Source: CAD feature listing. Evaluate the final solid. Frame: model axes, mm. A direction names the side the tool comes from. Round coordinates to 2 decimals unless told otherwise and drop trailing zeros. Write each loop counter-clockwise with the first axis right and the second up, starting at its lowest first coordinate (ties: lowest second). Pieces come first, ordered by that corner, then holes. Notation, with made-up numbers: M -12,39.25 L 13,39.25 A21 cw 13,66.25 Z; hole C 34.25,-3.75 d6. An arc over 180 degrees is marked long. Answer in a Markdown table with one row per item.
from build123d import *

# Parameters (mm, degrees)
EXTRUDE_1_DEPTH          = 9
EXTRUDE_2_DEPTH          = 5
FILLET_1_R               = 3.2
SKETCH_5_R               = 1.5
CUT_EXTRUDE_1_DEPTH      = 18
PATTERN_CIRCULAR_1_COUNT = 3
FILLET_2_R               = 3
EXTRUDE_START            = 50
EXTRUDE_3_DEPTH          = 50
FILLET_3_R               = 3


with BuildPart() as part:
    # 草图1 → 凸台-拉伸1 (new body)
    with BuildSketch(Plane(origin=(0, 0, 0), x_dir=(1, 0, 0), z_dir=(0, 1, 0))):
        Polygon((0, 22), (-19.052558883, -11), (19.052558883, -11), align=None)
        Polygon((0, 12), (-10.392304845, -6), (10.392304845, -6), align=None, mode=Mode.SUBTRACT)
    extrude(amount=EXTRUDE_1_DEPTH)

    # 草图3 → 凸台-拉伸2 (add)
    with BuildSketch(Plane(origin=(0, 9, 0), x_dir=(1, 0, 0), z_dir=(0, 1, 0))):
        Polygon((0, 28), (-24.248711306, -14), (24.248711306, -14), align=None)
        Polygon((0, 12), (-10.392304845, -6), (10.392304845, -6), align=None, mode=Mode.SUBTRACT)
    extrude(amount=EXTRUDE_2_DEPTH)

    # 圆角1
    fillet_1_edges = [part.edges().sort_by_distance(p)[0] for p in [
        (19.052558883, 4.5, 11),
        (-19.052558883, 4.5, 11),
        (0, 4.5, -22),
    ]]
    fillet(fillet_1_edges, radius=FILLET_1_R)

    # 草图5 → 切除-拉伸1 (cut)
    with BuildSketch(Plane(origin=(7, -46, 0), x_dir=(0, 0, -1), z_dir=(1, 0, 0))):
        with Locations((15, 50)):
            Circle(SKETCH_5_R)
    cut_extrude_1 = extrude(amount=-CUT_EXTRUDE_1_DEPTH, mode=Mode.SUBTRACT)

    # 阵列(圆周)1: 切除-拉伸1 ×3 about axis
    pattern_circular_1_axis = Axis((0, 0, 0), (0, 1, 0))
    for i in range(1, PATTERN_CIRCULAR_1_COUNT):
        add(cut_extrude_1.rotate(pattern_circular_1_axis, i * 360 / PATTERN_CIRCULAR_1_COUNT), mode=Mode.SUBTRACT)

    # 圆角2
    fillet_2_edges = [part.edges().sort_by_distance(p)[0] for p in [
        (24.248711306, 11.5, 14),
        (0, 11.5, -28),
        (-24.248711306, 11.5, 14),
    ]]
    fillet(fillet_2_edges, radius=FILLET_2_R)

    # 草图6 → 凸台-拉伸3 (add)
    with BuildSketch(Plane(origin=(0, 14, 0), x_dir=(1, 0, 0), z_dir=(0, 1, 0)).offset(EXTRUDE_START)):
        with BuildLine():
            Line((-2.598076211, 23.5), (-21.650635095, -9.5))
            ThreePointArc((-21.650635095, -9.5), (-21.650635095, -12.5), (-19.052558883, -14))
            Line((-19.052558883, -14), (19.052558883, -14))
            ThreePointArc((19.052558883, -14), (21.650635095, -12.5), (21.650635095, -9.5))
            Line((21.650635095, -9.5), (2.598076211, 23.5))
            ThreePointArc((2.598076211, 23.5), (0, 25), (-2.598076211, 23.5))
        make_face()
        Polygon((0, 20), (-17.320508076, -10), (17.320508076, -10), align=None, mode=Mode.SUBTRACT)
    extrude(amount=-EXTRUDE_3_DEPTH)

    # 圆角3
    fillet_3_edges = [part.edges().sort_by_distance(p)[0] for p in [
        (8.660254038, 14, -5),
        (-8.660254038, 14, -5),
        (0, 14, 10),
        (0, 39, -20),
        (-17.320508076, 39, 10),
        (17.320508076, 39, 10),
    ]]
    fillet(fillet_3_edges, radius=FILLET_3_R)


solid = part.part
Q1. Section A-A (y = 57). Return loops of the section in (x, z).
Solutions:
| item | result |
|---|---|
| outline | M -21.65,9.5 L -2.6,-23.5 A3 ccw 2.6,-23.5 L 21.65,9.5 A3 ccw 19.05,14 L -19.05,14 A3 ccw Z; hole M -14.72,5.5 L -2.6,-15.5 A3 ccw 2.6,-15.5 L 14.72,5.5 A3 ccw 12.12,10 L -12.12,10 A3 ccw Z |
Q2. Access query for faces 1 (the flat face through (9.62, 4.44, -5.34)), 2 (the flat face through (11.33, 9, -2.7)), 3 (the cylindrical face through (7.83, 14.9, -4.72)). Directions: +Z, -Z, +X, -X, +Y, -Y. A direction counts if a zero-diameter tool reaches every point of the face in a straight line with its end or side. Return the directions, or none.
Solutions:
| item | result |
|---|---|
| face 1 | -Z, +X, -Y |
| face 2 | -Y |
| face 3 | +Y |
Q3. Pull-direction query (Z, two-part tool) for faces 4 (the flat face through (0, 37, 14)), 5 (the cylindrical face through (16.26, 4.56, 9.44)), 6 (the cylindrical face through (14.7, 40.17, 8.54)), 7 (the flat face through (-9.432, 4.437, -5.664)); classes: pulls with the +Z half, pulls with the -Z half, needs draft (parallel to the pull), parting line crosses it, or undercut.
Solutions:
| item | result |
|---|---|
| face 4 | pulls with the +Z half |
| face 5 | parting line crosses it |
| face 6 | undercut |
| face 7 | pulls with the -Z half |
Q4. Section B-B (y = 4). Return loops of the section in (x, z).
Solutions:
| item | result |
|---|---|
| outline | M -16.28,6.2 L -15.88,5.5 L -12.7,11 L -13.51,11 A3.2 ccw Z; M -14.15,2.5 L -4.91,-13.5 L 4.91,-13.5 L 14.15,2.5 L 9.24,11 L -9.24,11 Z; M -3.18,-16.5 L -2.77,-17.2 A3.2 ccw 2.77,-17.2 L 3.18,-16.5 Z; M 12.7,11 L 15.88,5.5 L 16.28,6.2 A3.2 ccw 13.51,11 Z; hole M -10.39,6 L 0,-12 L 10.39,6 Z |
Q5. Material intervals for probe 1 along Z at (x, y) = (-0.25, 4); probe 2 along Z at (x, y) = (0, 22.5); probe 3 along Z at (x, y) = (2.75, 4), sorted ascending.
Solutions:
| item | result |
|---|---|
| probe 1 | z = -18.79 to -16.5, -13.5 to -11.57, 6 to 11 |
| probe 2 | z = -25 to -17, 10 to 14 |
| probe 3 | z = -17.24 to -16.5, -13.5 to -7.24, 6 to 11 |
Q6. Contact query for flat-ended pins moving along their axis: pin 1 Ø1 at (y, z) = (32.5, -17.5) entering from +X; pin 2 Ø12 at (y, z) = (40.5, -20) entering from +X; pin 3 Ø12 at (x, y) = (10.5, 50.5) entering from -Z. Output: stop coordinate, or through.
Solutions:
| item | result |
|---|---|
| pin 1 | stops at x = 6.35 |
| pin 2 | stops at x = 8.08 |
| pin 3 | stops at z = -20.21 |
